Source: CAD feature listing. Evaluate the final solid. Frame: model axes, mm. A direction names the side the tool comes from. Coordinates: 2 decimals unless noted, no trailing zeros. Write each loop counter-clockwise with the first axis right and the second up, starting at its lowest first coordinate (ties: lowest second). Pieces come first, ordered by that corner, then holes. Notation, with made-up numbers: (84.5, 28) -> (107.5, 28) arc R29 ccw to (107.5, 56) -> close; hole circle Ø4 at (81.25, 31.5). An arc over 180 degrees is marked (long way). Write item = value, one per line.
from build123d import *

# Parameters (mm, degrees)
SKETCH1_W                    = 38.1
SKETCH1_H                    = 101.6
BOSS_EXTRUDE1_DEPTH          = 12.7
SKETCH12_W                   = 5.8382662
SKETCH12_H                   = 3.81
CUT_EXTRUDE1_DEPTH           = 110.249530891
FILLET2_R                    = 1.27
F_10_0_1935_DIAMETER_HOLE2_D = 4.9784


with BuildPart() as part:
    # Sketch1 → Boss-Extrude1 (new body)
    with BuildSketch(Plane(origin=(0, 0, 0), x_dir=(1, 0, 0), z_dir=(0, 1, 0))):
        with Locations((19.05, 50.8)):
            Rectangle(SKETCH1_W, SKETCH1_H)
    extrude(amount=BOSS_EXTRUDE1_DEPTH)

    # Sketch12 → Cut-Extrude1 (cut, through all)
    with BuildSketch(Plane.ZY):
        with Locations((-72.8347159, 1.905)):
            Rectangle(SKETCH12_W, SKETCH12_H)
        with Locations((-28.8219007, 1.905)):
            Rectangle(SKETCH12_W, SKETCH12_H)
    extrude(amount=-CUT_EXTRUDE1_DEPTH, mode=Mode.SUBTRACT)

    # Fillet2
    fillet2_edges = [part.edges().sort_by_distance(p)[0] for p in [
        (19.05, 12.7, -101.6),
        (0, 12.7, -50.8),
        (19.05, 12.7, 0),
        (0, 6.35, 0),
        (0, 6.35, -101.6),
        (38.1, 6.35, -101.6),
        (38.1, 6.35, 0),
        (38.1, 12.7, -50.8),
    ]]
    fillet(fillet2_edges, radius=FILLET2_R)

    # #10 (0.1935) Diameter Hole2 (through all)
    with Locations(Plane(origin=(0, 12.7, 0), x_dir=(1, 0, 0), z_dir=(0, 1, 0))):
        with Locations((19.05, 95.25), (19.05, 6.35)):
            Hole(F_10_0_1935_DIAMETER_HOLE2_D / 2)


solid = part.part
1) Reachability of faces 1 (the flat face through (19, 2, -25.903)), 2 (the flat face through (0, 6, -50)) from +Z, -Z, +X, -X, +Y, -Y: full face, straight path, thin tool, end or side. Return the list, or none.
Answer block:
face_1 = +X, -X, -Y
face_2 = +Z, -Z, -X, +Y, -Y
2) Pull-direction query (X, two-part tool) for faces 3 (the cylindrical face through (21.537, 6.261, -6.459)), 4 (the flat face through (38.1, 6, -50)), 5 (the flat face through (19, 2, -69.916)); classes: +X half, -X half, draft (parallel to the pull), parting line (faces both ways), or undercut.
Answer block:
face_3 = undercut
face_4 = +X half
face_5 = draft
3) Material intervals for probe 1 along Z at (x, y) = (19.05, 5.25); probe 2 along Z at (x, y) = (34.5, 3); probe 3 along Z at (x, y) = (19.05, 3.5), sorted ascending. Write a range as [from, to].
Answer block:
probe_1 = [-101.6, -97.74], [-92.76, -8.84], [-3.86, 0]
probe_2 = [-101.6, -75.75], [-69.92, -31.74], [-25.9, 0]
probe_3 = [-101.6, -97.74], [-92.76, -75.75], [-69.92, -31.74], [-25.9, -8.84], [-3.86, 0]
4) Cut plane D-D, the plane z = -73.5. Output: boundary loops of the cut face in (x, y), and give its area (3 significant figures).
Answer block:
outline = (0, 3.81) -> (38.1, 3.81) -> (38.1, 11.43) arc R1.27 ccw to (36.83, 12.7) -> (1.27, 12.7) arc R1.27 ccw to (0, 11.43) -> close
area = 338 mm2
5) Cut plane B-B, the plane z = -6.35. Output: boundary loops of the cut face in (x, y).
Answer block:
outline = (0, 0) -> (16.56, 0) -> (16.56, 12.7) -> (1.27, 12.7) arc R1.27 ccw to (0, 11.43) -> close; (21.54, 0) -> (38.1, 0) -> (38.1, 11.43) arc R1.27 ccw to (36.83, 12.7) -> (21.54, 12.7) -> close
6) Cut plane A-A, the plane x = 19.05. Output: boundary loops of the cut face in (y, z), and give its area (3 significant figures).
Answer block:
outline = (0, -101.6) -> (11.43, -101.6) arc R1.27 ccw to (12.7, -100.33) -> (12.7, -97.74) -> (0, -97.74) -> close; (0, -92.76) -> (12.7, -92.76) -> (12.7, -8.84) -> (0, -8.84) -> (0, -25.9) -> (3.81, -25.9) -> (3.81, -31.74) -> (0, -31.74) -> (0, -69.92) -> (3.81, -69.92) -> (3.81, -75.75) -> (0, -75.75) -> close; (0, -3.86) -> (12.7, -3.86) -> (12.7, -1.27) arc R1.27 ccw to (11.43, 0) -> (0, 0) -> close
area = 1,120 mm2
7) First-contact query: pin 1 Ø1.8 at (x, z) = (16.5, -72) entering from -Y. Flat tip, straight axial feed; report the tip coordinate or a pass-through.
Answer block:
pin_1 = 3.81
8) Cut plane C-C, the plane x = 13. Output: boundary loops of the cut face in (y, z).
Answer block:
outline = (0, -101.6) -> (11.43, -101.6) arc R1.27 ccw to (12.7, -100.33) -> (12.7, -1.27) arc R1.27 ccw to (11.43, 0) -> (0, 0) -> (0, -25.9) -> (3.81, -25.9) -> (3.81, -31.74) -> (0, -31.74) -> (0, -69.92) -> (3.81, -69.92) -> (3.81, -75.75) -> (0, -75.75) -> close
